The model under review builds one solid part; all positions refer to its coordinate system, in mm. A direction names the side the tool comes from. Coordinates: 2 decimals unless noted, no trailing zeros. Loops run counter-clockwise (first coordinate to the right, second up) from the corner with the lowest first, then second, coordinate; pieces in that order, holes last. Notation, with made-up numbers: M 73,80.25 L 78,80.25 A19 cw 78,115.25 Z; hole C 16,57 d7. An arc over 180 degrees is marked long. Write item = value, one per line. Start each with the question number.
Q1. For faces 4 (the face through (6.466, -2.681, 6.437)), 5 (the face through (-4, 4, 12)), list the 3-axis set-ups (+Z, -Z, +X, -X, +Y, -Y) from which the entire face can be reached by the end or side of a thin tool; tool diameter is ignored.
Q2. Wall thickness on probe 1 along Y at (x, z) = (0, 8.25); probe 2 along Z at (x, y) = (17.5, -12); probe 3 along Y at (x, z) = (-2, 9.75): over which ranges is each line inside the solid? List them lowest first.
Q3. Clearance check with flat-ended pins moving along their axes: pin 1 Ø12 at (x, y) = (32.5, -19.5) entering from +Z; pin 2 Ø10.5 at (x, y) = (0, 0) entering from -Z; pin 3 Ø1.5 at (y, z) = (-13.5, 2.5) entering from -X; pin 4 Ø4 at (x, z) = (1, 6) entering from -Y. State where each tip first meets the part, or that it passes through.
Q4. We need section C-C on z = 7. Give the boundary of the cut face in (x, y).
Q5. We need section D-D on y = 15.5. Give the boundary of the cut face in (x, z).
Q6. We need section A-A on y = 0. Give the boundary of the cut face in (x, z), and give its area (3 significant figures).
Q7. Mouldability with a two-part tool opening along X and no side actions: class faces 1 (the face through (-1, -9, 0)), 2 (the face through (20.765, -39.923, 0.986)), 3 (the face through (-0.867, -3.905, 5.423)) as released by +X, released by -X, zero draft, split by the parting line, or undercut.
from build123d import *

# Parameters (mm, degrees)
SKETCH_R        = 45
SKETCH_R_2      = 4
PAD_DEPTH       = 2
SKETCH001_R     = 7
SKETCH001_R_2   = 4
PAD001_DEPTH    = 10
CHAMFER_SIZE    = 1
CHAMFER001_SIZE = 1


with BuildPart() as part:
    # Sketch → Pad (new body)
    with BuildSketch(Plane.XY):
        Circle(SKETCH_R)
        Circle(SKETCH_R_2, mode=Mode.SUBTRACT)
    extrude(amount=PAD_DEPTH)

    # Sketch001 (on Face4 of Pad) → Pad001 (join)
    with BuildSketch(Plane.XY.offset(2)):
        Circle(SKETCH001_R)
        Circle(SKETCH001_R_2, mode=Mode.SUBTRACT)
    extrude(amount=PAD001_DEPTH)

    # Chamfer
    chamfer_edges = [part.edges().sort_by_distance(p)[0] for p in [
        (-4, 0, 12),
    ]]
    chamfer(chamfer_edges, length=CHAMFER_SIZE)

    # Chamfer001
    chamfer001_edges = [part.edges().sort_by_distance(p)[0] for p in [
        (-7, 0, 12),
    ]]
    chamfer(chamfer001_edges, length=CHAMFER001_SIZE)


solid = part.part
Returned:
q1.face_4 = +Z
q1.face_5 = +Z, +X, -X, +Y, -Y
q2.probe_1 = -7 to -4, 4 to 7
q2.probe_2 = 0 to 2
q2.probe_3 = -6.71 to -3.46, 3.46 to 6.71
q3.pin_1 = 2
q3.pin_2 = 0
q3.pin_3 = -43.1
q3.pin_4 = -7
q4.outline = C 0,0 d14; hole C 0,0 d8
q5.outline = M -42.25,0 L 42.25,0 L 42.25,2 L -42.25,2 Z
q6.outline = M -45,0 L -4,0 L -4,11 L -5,12 L -6,12 L -7,11 L -7,2 L -45,2 Z; M 4,0 L 45,0 L 45,2 L 7,2 L 7,11 L 6,12 L 5,12 L 4,11 Z
q6.area = 222 mm^2
q7.face_1 = zero draft
q7.face_2 = split by the parting line
q7.face_3 = undercut
